Autodesk Inventor part; units mm, degrees
ref_plane "YZ Plane" through (0, 0, 0) normal (1, 0, 0) x (0, 1, 0)
ref_plane "XZ Plane" through (0, 0, 0) normal (0, 1, 0) x (-1, 0, 0)
ref_plane "XY Plane" through (0, 0, 0) normal (0, 0, 1) x (1, 0, 0)
sketch "Sketch1" plane through (0, 0, 0) normal (0, 0, 1) x (1, 0, 0)
  circle A0 centre (49.1868, 0) radius 3.175
  arc A1 (50.1181, 39.1289) -> (50.1181, 37.0464) centre (49.1868, 38.0877) ccw
  line L0 (49.1868, 38.0877) -> (49.1868, 0) construction
  line L1 (42.8368, 38.0877) -> (42.8368, 0)
  line L2 (55.5368, 0) -> (55.5368, 38.0877)
  arc A2 (55.5368, 38.0877) -> (42.8368, 38.0877) centre (49.1868, 38.0877) ccw
  arc A3 (42.8368, 0) -> (55.5368, 0) centre (49.1868, 0) ccw
  line L3 (47.7898, 38.0877) -> (50.3298, 38.0877) construction
  line L4 (50.1181, 37.0464) -> (50.1181, 39.1289)
  point P0 (49.1868, 19.0438)
  dimension "d0" = 12.7
  dimension "d3" = 2.794
  dimension "d4" = 2.54
extrude "Extrusion1" add sketch "Sketch1" along normal blind 3.175
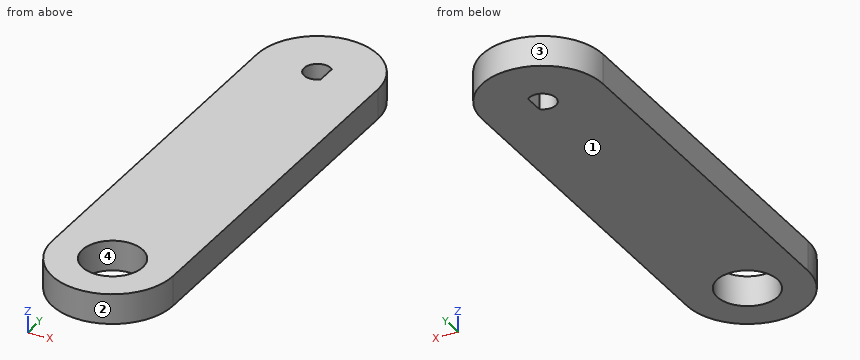
Geometry check sheet. Reference: the model listing, model coordinates, mm. Face numbers are marked on the shaded views. Round coordinates to 2 decimals unless told otherwise and drop trailing zeros. Order: outer loops, then holes, each group sorted by start corner. A loop starts at its lowest first (then second) coordinate and runs counter-clockwise, first axis right, second up. Notation, with made-up numbers: (-37.75, 64.25) -> (-13.75, 64.25) arc R12 cw to (-13.75, 75.25) -> close; hole circle Ø11 at (61, -34.5). An arc over 180 degrees is marked (long way). Return JSON: item names as keys, results as strings. Group by question number.
Q1. Section check D-D, the plane x = 45. Record the boundary of the cut face in (y, z) (3 decimals).
Q2. Section check A-A, the plane z = 0.65. Record the boundary of the cut face in (x, y) (3 decimals).
Q3. Material ranges on probe 1 along Y at (x, z) = (49.25, 1.3); probe 2 along Y at (x, z) = (48.75, 0.55); probe 3 along Y at (x, z) = (51.25, 0.4), recorded low to high. Write a range as from..to.
Q4. Gauge pin test, flat ends, axial feed: pin 1 (1 mm diameter, centred on y = -1, z = 1, fed in from +X); pin 2 (4.5 mm diameter, centred on x = 49.19, y = 38.09, fed in from -Z). Record the tip position at first contact, or that the pin passes through.
Q5. Release check for a two-part mould opening along Y. For the marked faces 1, 2, 3 and 4 record: released by +Y, released by -Y, zero draft, split by the parting line, or undercut.
Q6. Section check C-C, the plane y = -2.5. Record the boundary of the cut face in (x, z) (3 decimals), plus the area to 3 significant figures.
Q7. Section check B-B, the plane x = 48.25. Record the boundary of the cut face in (y, z) (3 decimals).
Numbers:
{
 "1": {"outline": "(-4.774, 0) -> (42.862, 0) -> (42.862, 3.175) -> (-4.774, 3.175) -> close"},
 "2": {"outline": "(42.837, 0) arc R6.35 ccw to (55.537, 0) -> (55.537, 38.088) arc R6.35 ccw to (42.837, 38.088) -> close; hole circle Ø6.35 at (49.187, 0); hole (50.118, 37.046) -> (50.118, 39.129) arc R1.397 ccw (long way) to start"},
 "3": {"probe 1": "-6.35..-3.17, 3.17..36.69, 39.48..44.44", "probe 2": "-6.33..-3.14, 3.14..36.76, 39.41..44.42", "probe 3": "-6.01..-2.41, 2.41..44.09"},
 "4": {"pin 1": "x = 55.52", "pin 2": "z = 0"},
 "5": {"face 1": "zero draft", "face 2": "released by -Y", "face 3": "released by +Y", "face 4": "undercut"},
 "6": {"outline": "(43.35, 0) -> (47.23, 0) -> (47.23, 3.175) -> (43.35, 3.175) -> close; (51.144, 0) -> (55.024, 0) -> (55.024, 3.175) -> (51.144, 3.175) -> close", "area": "24.6 mm^2"},
 "7": {"outline": "(-6.281, 0) -> (-3.034, 0) -> (-3.034, 3.175) -> (-6.281, 3.175) -> close; (3.034, 0) -> (37.051, 0) -> (37.051, 3.175) -> (3.034, 3.175) -> close; (39.124, 0) -> (44.368, 0) -> (44.368, 3.175) -> (39.124, 3.175) -> close"}
}
